Part model, mm, in its own coordinate system. A direction names the side the tool comes from. Give positions to 0.01 mm unless a question says otherwise; leave off trailing zeros. Write each loop counter-clockwise with the first axis right and the second up, starting at its lowest first coordinate (ties: lowest second). Pieces come first, ordered by that corner, then holes. Notation, with made-up numbers: (3, 11.25) - (14, 11.25) arc R24 cw to (14, 25.25) - close; hole circle Ø11 at (31.25, 56.5). An arc over 180 degrees is marked (long way). Answer in a Markdown table with one row per item. Add a question column.
1. Which spindle directions (+Z, -Z, +X, -X, +Y, -Y) get a long thin tool onto all of the face, cutting with end or side? Do faces 4 (the flat face through (-13, 4.826, 27)), 5 (the flat face through (-48, 4.826, -8)), 6 (the flat face through (-68.066, -15, 10)). Say none if no direction does.
2. Pull direction X, two halves, no side cores. Call faces 1 (the flat face through (-55, -11, 22.555)), 2 (the flat face through (-43.116, -10, 35)), 3 (the flat face through (0, 6, 10)): released by +X, released by -X, zero draft, split by the parting line, or undercut.
3. Band-saw the part on D-D on x = -16. Write the cut outline in (y, z), plus the area to 3 significant figures.
4. Probe line 1 along Z through (x, y) = (-30.5, -3); line 2 along Z through (x, y) = (-44.5, -2); line 3 along Z through (x, y) = (5.5, 3). List the from-to ranges inside material, lowest first.
5. Band-saw the part on A-A on y = -4.5. Write the cut outline in (x, z), plus the area to 3 significant figures.
6. Band-saw the part on B-B on x = -32. Write the cut outline in (y, z), plus the area to 3 significant figures.
7. Band-saw the part on C-C on z = 41. Write the cut outline in (x, y), plus the area to 3 significant figures.
8. Drop flat-ended pins along their axis: pin 1 Ø12 at (x, y) = (-40.5, -21.5) entering from -Z; pin 2 Ø6 at (x, y) = (-25, -16) entering from -Z; pin 3 Ø3.5 at (x, z) = (4.5, 15.5) entering from -Y. Give the stop position or say it passes through.
```python
from build123d import *

# Parameters (mm, degrees)
SKETCH1_W           = 54.737
SKETCH1_H           = 25.4
SKETCH1_W_2         = 40.2717
SKETCH1_H_2         = 19.7104
BOSS_EXTRUDE2_DEPTH = 9.906
SKETCH3_R           = 9.8552
SKETCH3_R_2         = 5.461
BOSS_EXTRUDE3_DEPTH = 0.508
SKETCH9_W           = 7.23265
SKETCH9_H           = 1.27
CUT_EXTRUDE2_DEPTH  = 5.08
SKETCH12_W          = 54.737
SKETCH12_H          = 2.8448
BOSS_EXTRUDE4_DEPTH = 30.734
BOSS_EXTRUDE5_DEPTH = 20.5613
BOSS_EXTRUDE6_DEPTH = 24.94915
BOSS_EXTRUDE7_DEPTH = 24.94915
BOSS_EXTRUDE8_DEPTH = 40.64
BOSS_EXTRUDE9_DEPTH = 5.08
SKETCH25_W          = 2.54
SKETCH25_H          = 6.35
CUT_EXTRUDE3_DEPTH  = 2.54


with BuildPart() as part:
    # Sketch1 → Boss-Extrude2 (new body)
    with BuildSketch(Plane(origin=(0, 0, 0), x_dir=(1, 0, 0), z_dir=(0, 1, 0))):
        with Locations((-20.13585, -9.8552)):
            Rectangle(SKETCH1_W, SKETCH1_H)
        with Locations((-20.13585, -9.8552)):
            Rectangle(SKETCH1_W_2, SKETCH1_H_2, mode=Mode.SUBTRACT)
    extrude(amount=BOSS_EXTRUDE2_DEPTH)

    # Sketch3 → Boss-Extrude3 (add)
    with BuildSketch(Plane(origin=(0, 9.906, 0), x_dir=(1, 0, 0), z_dir=(0, 1, 0))):
        with Locations((-30.4165, -9.8552)):
            Circle(SKETCH3_R)
        with Locations((-30.4165, -9.8552)):
            Circle(SKETCH3_R_2, mode=Mode.SUBTRACT)
        with BuildLine():
            ThreePointArc((-30.4165, -19.7104), (-37.38517875, -16.82387875), (-40.2717, -9.8552))
            Line((-40.2717, -9.8552), (-40.2717, -19.7104))
            Line((-40.2717, -19.7104), (-30.4165, -19.7104))
        make_face()
        with BuildLine():
            Line((0, 0), (-30.4165, 0))
            ThreePointArc((-30.4165, 0), (-23.44782125, -2.88652125), (-20.5613, -9.8552))
            ThreePointArc((-20.5613, -9.8552), (-23.44782125, -16.82387875), (-30.4165, -19.7104))
            Line((-30.4165, -19.7104), (0, -19.7104))
            Line((0, -19.7104), (0, 0))
        make_face()
        with BuildLine():
            Line((-30.4165, 0), (-40.2717, 0))
            Line((-40.2717, 0), (-40.2717, -9.8552))
            ThreePointArc((-40.2717, -9.8552), (-37.38517875, -2.88652125), (-30.4165, 0))
        make_face()
    extrude(amount=-BOSS_EXTRUDE3_DEPTH)

    # Sketch9 → Cut-Extrude2 (cut)
    with BuildSketch(Plane.XZ):
        with Locations((-43.888025, 9.8552)):
            Rectangle(SKETCH9_W, SKETCH9_H)
        with Locations((3.616325, 9.8552)):
            Rectangle(SKETCH9_W, SKETCH9_H)
    extrude(amount=-CUT_EXTRUDE2_DEPTH, mode=Mode.SUBTRACT)

    # Sketch12 → Boss-Extrude4 (add)
    with BuildSketch(Plane.XZ):
        with Locations((-20.13585, 21.1328)):
            Rectangle(SKETCH12_W, SKETCH12_H)
        with Locations((-20.13585, -1.4224)):
            Rectangle(SKETCH12_W, SKETCH12_H)
    extrude(amount=BOSS_EXTRUDE4_DEPTH)

    # Sketch19 → Boss-Extrude5 (add)
    with BuildSketch(Plane.ZY.offset(47.50435)):
        Polygon((-2.8448, -30.734), (0, -30.734), (0, 0), (19.7104, 0), (19.7104, -30.734), (22.5552, -30.734), (22.5552, 9.906), (-2.8448, 9.906), align=None)
    extrude(amount=BOSS_EXTRUDE5_DEPTH)

    # Sketch20 → Boss-Extrude6 (add)
    with BuildSketch(Plane(origin=(0, 0, -2.8448), x_dir=(-1, 0, 0), z_dir=(0, 0, -1))):
        Polygon((17.7165, 9.906), (43.1165, 9.906), (43.1165, -30.734), (40.3225, -30.734), (40.3225, 0), (20.5105, 0), (20.5105, -30.734), (17.7165, -30.734), align=None)
    extrude(amount=BOSS_EXTRUDE6_DEPTH)

    # Sketch21 → Boss-Extrude7 (add)
    with BuildSketch(Plane.XY.offset(22.5552)):
        Polygon((-43.1165, 9.906), (-43.1165, -30.734), (-40.3225, -30.734), (-40.3225, 0), (-20.5105, 0), (-20.5105, -30.734), (-17.7165, -30.734), (-17.7165, 9.906), align=None)
    extrude(amount=BOSS_EXTRUDE7_DEPTH)

    # Sketch23 → Boss-Extrude8 (add)
    with BuildSketch(Plane(origin=(0, 9.906, 0), x_dir=(1, 0, 0), z_dir=(0, 1, 0))):
        with BuildLine():
            Line((-68.06565, 2.8448), (-68.06565, -22.5552))
            ThreePointArc((-68.06565, -22.5552), (-70.149968207, -9.8552), (-68.06565, 2.8448))
        make_face()
        with BuildLine():
            Line((-43.1165, -47.50435), (-17.7165, -47.50435))
            ThreePointArc((-17.7165, -47.50435), (-30.4165, -49.588668207), (-43.1165, -47.50435))
        make_face()
        with BuildLine():
            Line((7.23265, -22.5552), (7.23265, 2.8448))
            ThreePointArc((7.23265, 2.8448), (9.316968207, -9.8552), (7.23265, -22.5552))
        make_face()
        with BuildLine():
            Line((-17.7165, 27.79395), (-43.1165, 27.79395))
            ThreePointArc((-43.1165, 27.79395), (-30.4165, 29.878268207), (-17.7165, 27.79395))
        make_face()
    extrude(amount=-BOSS_EXTRUDE8_DEPTH)

    # Sketch24 → Boss-Extrude9 (add)
    with BuildSketch(Plane(origin=(0, 9.906, 0), x_dir=(1, 0, 0), z_dir=(0, 1, 0))):
        with BuildLine():
            ThreePointArc((-43.1165, 15.319375), (-50.35451929, 10.08281929), (-55.591075, 2.8448))
            Line((-55.591075, 2.8448), (-43.1165, 2.8448))
            Line((-43.1165, 2.8448), (-43.1165, 15.319375))
        make_face()
        with BuildLine():
            ThreePointArc((-55.591075, -22.5552), (-50.35451929, -29.79321929), (-43.1165, -35.029775))
            Line((-43.1165, -35.029775), (-43.1165, -22.5552))
            Line((-43.1165, -22.5552), (-55.591075, -22.5552))
        make_face()
        with BuildLine():
            ThreePointArc((-17.7165, -35.029775), (-10.47848071, -29.79321929), (-5.241925, -22.5552))
            Line((-5.241925, -22.5552), (-17.7165, -22.5552))
            Line((-17.7165, -22.5552), (-17.7165, -35.029775))
        make_face()
        with BuildLine():
            ThreePointArc((-5.241925, 2.8448), (-10.47848071, 10.08281929), (-17.7165, 15.319375))
            Line((-17.7165, 15.319375), (-17.7165, 2.8448))
            Line((-17.7165, 2.8448), (-5.241925, 2.8448))
        make_face()
    extrude(amount=-BOSS_EXTRUDE9_DEPTH)

    # Sketch25 → Cut-Extrude3 (cut)
    with BuildSketch(Plane.XZ.offset(30.734)):
        with Locations((-69.33565, 9.8552)):
            Rectangle(SKETCH25_W, SKETCH25_H)
    extrude(amount=-CUT_EXTRUDE3_DEPTH, mode=Mode.SUBTRACT)


solid = part.part
```
Values:
| question | item | result |
|---|---|---|
| 1 | face 4 | +Z, +X, -Y |
| 1 | face 5 | -Z, -X, -Y |
| 1 | face 6 | -Y |
| 2 | face 1 | zero draft |
| 2 | face 2 | released by -X |
| 2 | face 3 | undercut |
| 3 | outline | (-30.73, -2.84) - (4.83, -2.84) - (4.83, -14.38) - (9.91, -14.38) - (9.91, 34.09) - (4.83, 34.09) - (4.83, 22.56) - (-30.73, 22.56) - (-30.73, 19.71) - (9.4, 19.71) - (9.4, 0) - (-30.73, 0) - close |
| 3 | area | 358 mm² |
| 4 | line 1 | z = -29.88 to -27.79, -2.84 to 0, 19.71 to 22.56, 47.5 to 49.59 |
| 4 | line 2 | z = -2.84 to 0, 19.71 to 22.56 |
| 4 | line 3 | z = -2.84 to 9.22, 10.49 to 22.56 |
| 5 | outline | (-68.07, -2.84) - (-43.12, -2.84) - (-43.12, -27.79) arc R39.73 ccw to (-17.72, -27.79) - (-17.72, -2.84) - (7.23, -2.84) arc R39.73 ccw to (7.23, 22.56) - (-17.72, 22.56) - (-17.72, 47.5) arc R39.73 ccw to (-43.12, 47.5) - (-43.12, 22.56) - (-68.07, 22.56) arc R39.73 ccw to start; hole (-68.07, 0) - (7.23, 0) - (7.23, 19.71) - (-68.07, 19.71) - close; hole (-40.32, -27.79) - (-20.51, -27.79) - (-20.51, -2.84) - (-40.32, -2.84) - close; hole (-40.32, 22.56) - (-20.51, 22.56) - (-20.51, 47.5) - (-40.32, 47.5) - close |
| 5 | area | 849 mm² |
| 6 | outline | (-30.73, -29.85) - (9.91, -29.85) - (9.91, 4.63) - (9.4, 4.63) - (9.4, 0) - (-30.73, 0) - (-30.73, -2.84) - (0, -2.84) - (0, -27.79) - (-30.73, -27.79) - close; (-30.73, 19.71) - (9.4, 19.71) - (9.4, 15.08) - (9.91, 15.08) - (9.91, 49.56) - (-30.73, 49.56) - (-30.73, 47.5) - (0, 47.5) - (0, 22.56) - (-30.73, 22.56) - close |
| 6 | area | 897 mm² |
| 7 | outline | (-43.12, -30.73) - (-40.32, -30.73) - (-40.32, 0) - (-20.51, 0) - (-20.51, -30.73) - (-17.72, -30.73) - (-17.72, 9.91) - (-43.12, 9.91) - close |
| 7 | area | 423 mm² |
| 8 | pin 1 | stops at z = -29.67 |
| 8 | pin 2 | stops at z = -29.8 |
| 8 | pin 3 | stops at y = 0 |
